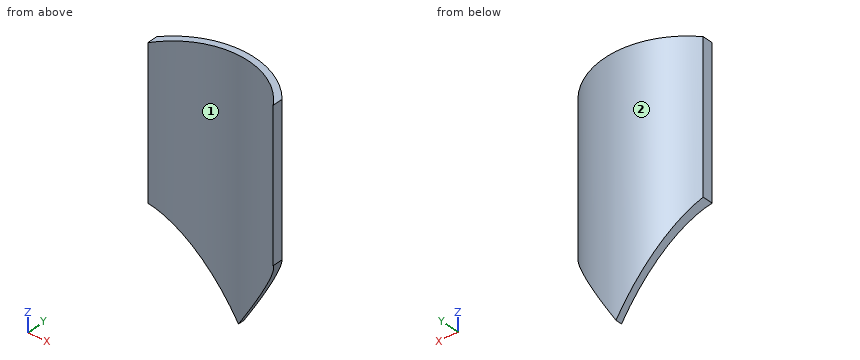
```python
from build123d import *

# Parameters (mm, degrees)
F1_DEPTH      = 250
F1_DEPTH_BACK = 250
F3_DEPTH      = 165.65046


with BuildPart() as f1:
    # F0 (on Top) → F1 (new body, two sides)
    with BuildSketch(Plane.XY) as f1_sk:
        with BuildLine():
            Line((125, 87.878756), (125, 108.695647))
            ThreePointArc((125, 108.695647), (0, 165.64946), (-125, 108.695647))
            Line((-125, 108.695647), (-125, 87.878756))
            ThreePointArc((-125, 87.878756), (0, 152.799463), (125, 87.878756))
        make_face()
    extrude(amount=F1_DEPTH)
    extrude(f1_sk.sketch, amount=-F1_DEPTH_BACK)

    # F2 (on Front) → F3 (cut, through all)
    with BuildSketch(Plane.XZ):
        Polygon((-125, -250.156015), (0, -250), (-125, -48.299942), align=None)
        Polygon((125, -250), (125, -48.299942), (0, -250), align=None)
    extrude(amount=-F3_DEPTH, mode=Mode.SUBTRACT)


solid = f1.part
```
Geometry check sheet. Reference: the model listing, model coordinates, mm. Face numbers are marked on the shaded views. Round coordinates to 2 decimals unless told otherwise and drop trailing zeros. Order: outer loops, then holes, each group sorted by start corner. A loop starts at its lowest first (then second) coordinate and runs counter-clockwise, first axis right, second up. Notation, with made-up numbers: (37, -30) -> (86, -30) arc R20 ccw to (86, -24) -> close; hole circle Ø4 at (-39.75, -35.5). An arc over 180 degrees is marked (long way). Return JSON: item names as keys, results as strings. Group by question number.
Q1. Release check for a two-part mould opening along X. For the marked faces 1 and 2 record: released by +X, released by -X, zero draft, split by the parting line, or undercut.
Q2. Section check A-A, the plane y = 127. Record the boundary of the cut face in (x, z), plus the area to 3 significant figures.
Q3. Section check D-D, the plane x = -7.5. Record the boundary of the cut face in (y, z), plus the area to 3 significant figures.
Q4. Material ranges on probe 1 along X at (y, z) = (98.5, -28.5); probe 2 along X at (y, z) = (108.5, 206); probe 3 along Y at (x, z) = (113.5, 211), recorded low to high. Write a range as from..to.
Q5. Section check B-B, the plane z = -13.5. Record the boundary of the cut face in (x, y), plus the area to 3 significant figures.
Q6. Section check C-C, the plane y = 98.5. Record the boundary of the cut face in (x, z), plus the area to 3 significant figures.
Q7. Gauge pin test, flat ends, axial feed: pin 1 (8 mm diameter, centred on y = 149.5, z = 124.5, fed in from -X); pin 2 (2 mm diameter, centred on y = 136, z = -50.5, fed in from +X); pin 3 (8 mm diameter, centred on x = 19.5, z = -189, fed in from +Y). Record the tip position at first contact, or that the pin passes through.
Numbers:
{
 "1": {"face 1": "undercut", "face 2": "split by the parting line"},
 "2": {"outline": "(-106.35, -78.39) -> (-84.96, -112.9) -> (-84.96, 250) -> (-106.35, 250) -> close; (84.96, -112.9) -> (106.35, -78.39) -> (106.35, 250) -> (84.96, 250) -> close", "area": "14,800 mm^2"},
 "3": {"outline": "(152.62, -237.9) -> (165.48, -237.9) -> (165.48, 250) -> (152.62, 250) -> close", "area": "6,280 mm^2"},
 "4": {"probe 1": "-125..-116.81, 116.81..125", "probe 2": "-125..-107.59, 107.59..125", "probe 3": "102.3..120.65"},
 "5": {"outline": "(-125, 87.88) arc R152.8 cw to (125, 87.88) -> (125, 108.7) arc R165.65 ccw to (-125, 108.7) -> close", "area": "3,700 mm^2"},
 "6": {"outline": "(-125, -48.3) -> (-116.81, -61.51) -> (-116.81, 250) -> (-125, 250) -> close; (116.81, -61.51) -> (125, -48.3) -> (125, 250) -> (116.81, 250) -> close", "area": "4,990 mm^2"},
 "7": {"pin 1": "x = -79.18", "pin 2": "x = 95.99", "pin 3": "y = 164.92"}
}
